```python
from build123d import *

# Parameters (mm, degrees)
SKETCH1_R                             = 9.525
BOSS_EXTRUDE1_DEPTH                   = 60.325
F_1_4_20_TAPPED_HOLE1_D               = 5.1054
F_1_4_20_TAPPED_HOLE1_DEPTH           = 16.51
F_1_4_20_TAPPED_HOLE1_TIP             = 1.533816902
F_1_4_20_TAPPED_HOLE1_ON_FACE_2_D     = 5.1054
F_1_4_20_TAPPED_HOLE1_ON_FACE_2_DEPTH = 16.51
F_1_4_20_TAPPED_HOLE1_ON_FACE_2_TIP   = 1.533816902


with BuildPart() as part:
    # Sketch1 → Boss-Extrude1 (new, symmetric)
    with BuildSketch(Plane(origin=(0, 0, 0), x_dir=(0, 0, -1), z_dir=(1, 0, 0))):
        with Locations(Location((0, 0, 0), (0, 0, 180))):
            Circle(SKETCH1_R)
    extrude(amount=BOSS_EXTRUDE1_DEPTH, both=True)

    # 1/4-20 Tapped Hole1
    with Locations(Plane(origin=(60.325, 0, 0), x_dir=(0, 0, 1), z_dir=(1, 0, 0))):
        with Locations((0, 0)):
            Hole(F_1_4_20_TAPPED_HOLE1_D / 2, depth=F_1_4_20_TAPPED_HOLE1_DEPTH)
            with Locations((0, 0, -(F_1_4_20_TAPPED_HOLE1_DEPTH + F_1_4_20_TAPPED_HOLE1_TIP / 2))):  # 118° drill point
                Cone(0, F_1_4_20_TAPPED_HOLE1_D / 2, F_1_4_20_TAPPED_HOLE1_TIP, mode=Mode.SUBTRACT)

    # 1/4-20 Tapped Hole1 on face 2
    with Locations(Plane(origin=(-60.325, 0, 0), x_dir=(0, 0, -1), z_dir=(-1, 0, 0))):
        with Locations((0, 0)):
            Hole(F_1_4_20_TAPPED_HOLE1_ON_FACE_2_D / 2, depth=F_1_4_20_TAPPED_HOLE1_ON_FACE_2_DEPTH)
            with Locations((0, 0, -(F_1_4_20_TAPPED_HOLE1_ON_FACE_2_DEPTH + F_1_4_20_TAPPED_HOLE1_ON_FACE_2_TIP / 2))):  # 118° drill point
                Cone(0, F_1_4_20_TAPPED_HOLE1_ON_FACE_2_D / 2, F_1_4_20_TAPPED_HOLE1_ON_FACE_2_TIP, mode=Mode.SUBTRACT)


solid = part.part
```
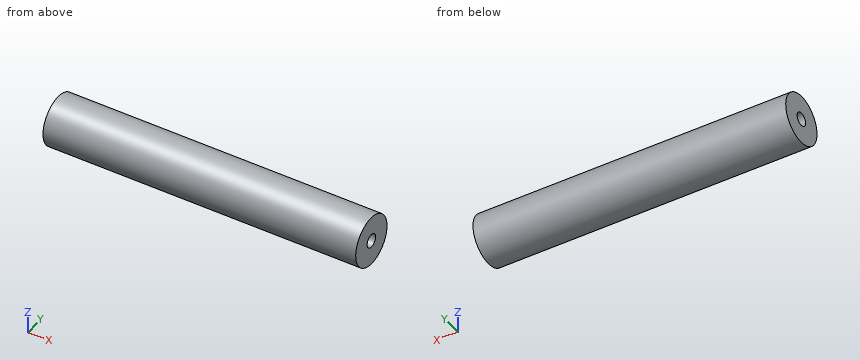
Can you work these out from the model? Positions are in its coordinate system, mm. Give positions to 0.01 mm unless a question says otherwise; leave off trailing zeros. Order: outer loops, then holes, each group sorted by start corner. A loop starts at its lowest first (then second) coordinate and runs counter-clockwise, first axis right, second up. Notation, with made-up numbers: M 83,45 L 138,45 A9 ccw 138,54 Z; hole C 13.25,17.5 d8. An arc over 180 degrees is marked long. Write item = value, one per line. Start each with the question number.
Q1. Will these pins go through, and if not, where does the flat tip stop? pin 1 Ø1.5 at (x, y) = (6, 3) entering from +Z; pin 2 Ø3 at (y, z) = (0, 0) entering from +X; pin 3 Ø3 at (x, z) = (-2, -5) entering from -Y.
Q2. Suppose I cut it at B-B (z = 7.5). Write out the boundary of the cut face in (x, y) (3 decimals), plus the area to 3 significant figures.
Q3. Suppose I cut it at A-A (x = -37). Write out the boundary of the cut face in (y, z) (3 decimals), plus the area to 3 significant figures.
Q4. I need wall thicknesses on probe 1 along Y at (x, z) = (-56, 0) (3 decimals); probe 2 along Y at (x, z) = (7, -0.5); probe 3 along Y at (x, z) = (-21, 4.75). Which ranges of each line are inside material? Lowest first, please. Write a range as [from, to].
Check result:
q1.pin_1 = 9.26
q1.pin_2 = 43.18
q1.pin_3 = -8.86
q2.outline = M -60.325,-5.872 L 60.325,-5.872 L 60.325,5.872 L -60.325,5.872 Z
q2.area = 1,420 mm2
q3.outline = C 0,0 d19.05
q3.area = 285 mm2
q4.probe_1 = [-9.525, -2.553], [2.553, 9.525]
q4.probe_2 = [-9.51, 9.51]
q4.probe_3 = [-8.26, 8.26]
